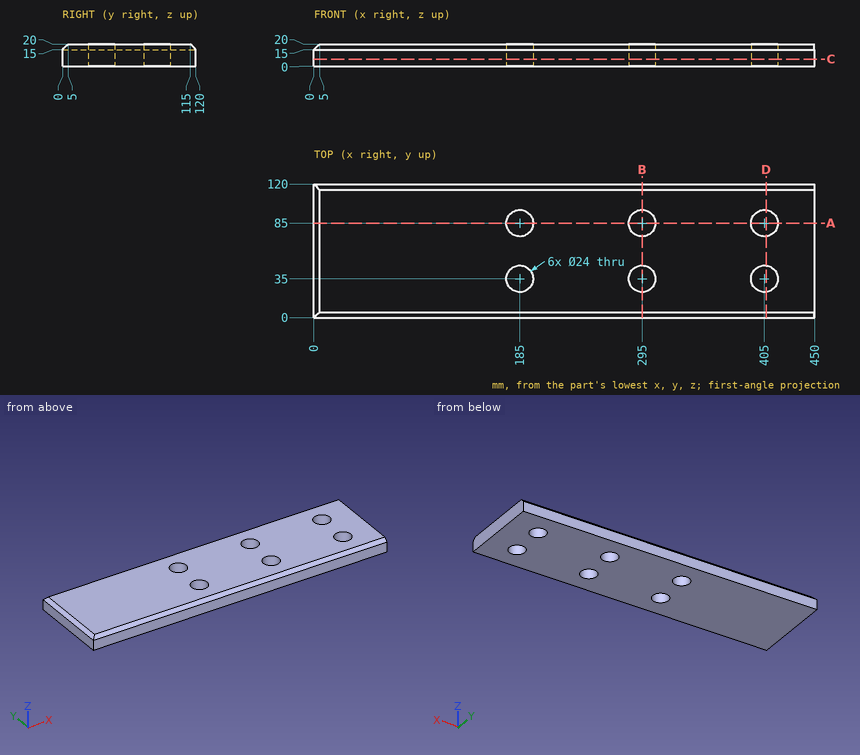
Answer from the drawing. Dimensions are ordinates in mm from the lowest x, y and z of the part. Coordinates: 2 decimals unless noted, no trailing zeros. Write each loop counter-clockwise with the first axis right and the second up, starting at its lowest first coordinate (ties: lowest second). Pieces come first, ordered by that corner, then holes. Notation, with made-up numbers: (4, 52.25) - (40, 52.25) arc R32 ccw to (40, 85.25) - close; hole circle Ø9 at (31, 2). An arc over 180 degrees is marked (long way). Return JSON: item names as keys, results as strings.
1. The part is cut by section D-D on x = 406.5. Determine the outline of the cut face in (y, z), then the cut area to 3 significant figures.
Final values:
{"outline": "(0, 0) - (23.09, 0) - (23.09, 20) - (5, 20) - (0, 15) - close; (46.91, 0) - (73.09, 0) - (73.09, 20) - (46.91, 20) - close; (96.91, 0) - (120, 0) - (120, 15) - (115, 20) - (96.91, 20) - close", "area": "1,420 mm^2"}
2. Consider line 1 along Y through (x, z) = (295, 10.5); line 2 along Y through (x, z) = (305.5, 12); line 3 along X through (y, z) = (30, 12). Determine where each line is inside the solid, lowest interval first.
Final values:
{"line 1": "0 to 23, 47 to 73, 97 to 120", "line 2": "0 to 29.19, 40.81 to 79.19, 90.81 to 120", "line 3": "0 to 174.09, 195.91 to 284.09, 305.91 to 394.09, 415.91 to 450"}
3. The part is cut by section C-C on z = 6.5. Determine the outline of the cut face in (x, y).
Final values:
{"outline": "(0, 0) - (450, 0) - (450, 120) - (0, 120) - close; hole circle Ø24 at (185, 35); hole circle Ø24 at (185, 85); hole circle Ø24 at (295, 35); hole circle Ø24 at (295, 85); hole circle Ø24 at (405, 35); hole circle Ø24 at (405, 85)"}
4. The part is cut by section B-B on x = 295. Determine the outline of the cut face in (y, z), then the cut area to 4 significant figures.
Final values:
{"outline": "(0, 0) - (23, 0) - (23, 20) - (5, 20) - (0, 15) - close; (47, 0) - (73, 0) - (73, 20) - (47, 20) - close; (97, 0) - (120, 0) - (120, 15) - (115, 20) - (97, 20) - close", "area": "1,415 mm^2"}
5. The part is cut by section A-A on y = 85. Determine the outline of the cut face in (x, z), then the cut area to 3 significant figures.
Final values:
{"outline": "(0, 0) - (173, 0) - (173, 20) - (5, 20) - (0, 15) - close; (197, 0) - (283, 0) - (283, 20) - (197, 20) - close; (307, 0) - (393, 0) - (393, 20) - (307, 20) - close; (417, 0) - (450, 0) - (450, 20) - (417, 20) - close", "area": "7,550 mm^2"}
